Geometry check sheet. Reference: the model listing, model coordinates, mm. A direction names the side the tool comes from. Coordinates: 2 decimals unless noted, no trailing zeros. Loops run counter-clockwise (first coordinate to the right, second up) from the corner with the lowest first, then second, coordinate; pieces in that order, holes last. Notation, with made-up numbers: (40, -6) - (93, -6) arc R22 ccw to (93, 19) - close; hole circle Ø7 at (9.5, 85). An arc over 180 degrees is marked (long way). One line per item, written item: value.
from build123d import *

# Parameters (mm, degrees)
BOSS_EXTRUDE1_DEPTH = 63.5
CUT_EXTRUDE1_DEPTH  = 151.804144505
SKETCH3_R           = 6.35
CUT_EXTRUDE2_DEPTH  = 175.596133978
SKETCH4_R           = 3.175
CUT_EXTRUDE3_DEPTH  = 175.596133978


with BuildPart() as part:
    # Sketch1 → Boss-Extrude1 (new body)
    with BuildSketch(Plane.XY):
        Polygon((12.7, -127), (50.8, -127), (50.8, 0), (-50.8, 0), (-50.8, -127), (-12.7, -127), (-12.7, -114.3), (12.7, -114.3), align=None)
    extrude(amount=-BOSS_EXTRUDE1_DEPTH)

    # Sketch2 → Cut-Extrude1 (cut, through all)
    with BuildSketch(Plane(origin=(0, 0, 0), x_dir=(1, 0, 0), z_dir=(0, 1, 0))):
        Polygon((-38.1, 50.8), (-38.1, 63.5), (38.1, 63.5), (38.1, 50.8), (38.1, 12.7), (-38.1, 12.7), align=None)
    extrude(amount=-CUT_EXTRUDE1_DEPTH, mode=Mode.SUBTRACT)

    # Sketch3 → Cut-Extrude2 (cut, through all)
    with BuildSketch(Plane.ZY.offset(50.8)):
        with Locations((-7.159845265, -35.322751873)):
            Circle(SKETCH3_R)
        with Locations((-7.159845265, -52.530231645)):
            Circle(SKETCH3_R)
        with Locations((-7.159845265, -71.0282724)):
            Circle(SKETCH3_R)
    extrude(amount=-CUT_EXTRUDE2_DEPTH, mode=Mode.SUBTRACT)

    # Sketch4 → Cut-Extrude3 (cut, through all)
    with BuildSketch(Plane.ZY.offset(50.8)):
        with Locations((-57.15, -120.65)):
            Circle(SKETCH4_R)
        with Locations((-44.45, -120.65)):
            Circle(SKETCH4_R)
        with Locations((-31.75, -120.65)):
            Circle(SKETCH4_R)
    extrude(amount=-CUT_EXTRUDE3_DEPTH, mode=Mode.SUBTRACT)


solid = part.part
(1) Material ranges on probe 1 along Z at (x, y) = (46.5, -120.5); probe 2 along X at (y, z) = (-73, -55); probe 3 along Y at (x, z) = (-47.75, -44.45) (3 decimals), recorded low to high. Write a range as from..to.
Reply:
probe 1: -63.5..-60.32, -53.98..-47.62, -41.28..-34.92, -28.58..0
probe 2: -50.8..-38.1, 38.1..50.8
probe 3: -127..-123.825, -117.475..0
(2) Cross-section at B-B on y = -9. Record the cut outline in (x, z), and give its area (3 significant figures).
Reply:
outline: (-50.8, -63.5) - (-38.1, -63.5) - (-38.1, -12.7) - (38.1, -12.7) - (38.1, -63.5) - (50.8, -63.5) - (50.8, 0) - (-50.8, 0) - close
area: 2,580 mm2
(3) Access from +Z, -Z, +X, -X, +Y, -Y to the whole of each face (thin tool, end or side, straight path). Record for faces 1 (the face through (-38.1, -63, -38)), 2 (the face through (-12.7, -121, -6)), 3 (the face through (-45, -63, -63.5)).
Reply:
face 1: -Z, +Y, -Y
face 2: +Z, -Z, -Y
face 3: -Z, +X, -X, +Y, -Y
(4) Cross-section at D-D on y = -120.65. State how many separate pieces and enclosed holes the cut face has, and give its area (3 significant figures).
Reply:
separate pieces: 8
enclosed holes: 0
area: 1,770 mm2
(5) Cross-section at C-C on x = 10. Record the cut outline in (y, z), and give its area (3 significant figures).
Reply:
outline: (-114.3, -12.7) - (-74.13, -12.7) arc R6.35 cw (long way) to (-67.93, -12.7) - (-55.63, -12.7) arc R6.35 cw (long way) to (-49.43, -12.7) - (-38.43, -12.7) arc R6.35 cw (long way) to (-32.22, -12.7) - (0, -12.7) - (0, 0) - (-114.3, 0) - close
area: 1,080 mm2
(6) Release check for a two-part mould opening along Y. For faces 4 (the face through (38.1, -63, -38)), 5 (the face through (-44.539, -123.467, -42.985)), 6 (the face through (1, 0, -10)) record: pulls with the +Y half, pulls with the -Y half, needs draft (parallel to the pull), parting line crosses it, or undercut.
Reply:
face 4: needs draft
face 5: undercut
face 6: pulls with the +Y half
(7) Cross-section at A-A on z = -44.45. Record the cut outline in (x, y) (3 decimals), and give its area (3 significant figures).
Reply:
outline: (-50.8, -127) - (-38.1, -127) - (-38.1, -123.825) - (-50.8, -123.825) - close; (-50.8, -117.475) - (-38.1, -117.475) - (-38.1, 0) - (-50.8, 0) - close; (38.1, -127) - (50.8, -127) - (50.8, -123.825) - (38.1, -123.825) - close; (38.1, -117.475) - (50.8, -117.475) - (50.8, 0) - (38.1, 0) - close
area: 3,060 mm2
(8) Go/stop test with a flat-tipped pin: pin 1 Ø3.5 at (x, y) = (8.5, -41) entering from -Z. Record where the tip stops, or that it passes through.
Reply:
pin 1: z = -12.7
